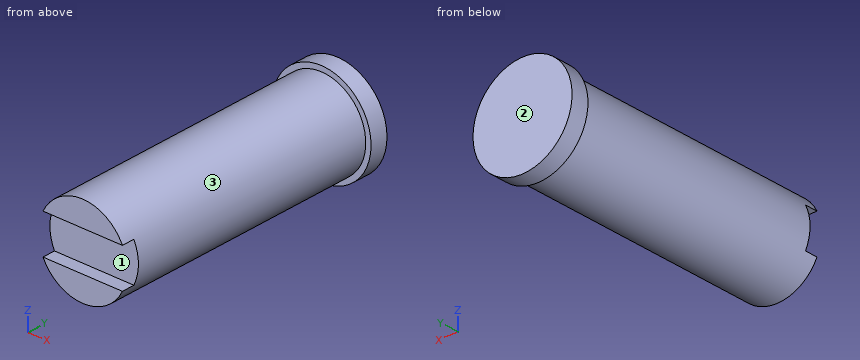
Autodesk Inventor part; units mm, degrees
ref_plane "YZ Plane" through (0, 0, 0) normal (1, 0, 0) x (0, 1, 0)
ref_plane "XZ Plane" through (0, 0, 0) normal (0, 1, 0) x (-1, 0, 0)
ref_plane "XY Plane" through (0, 0, 0) normal (0, 0, 1) x (1, 0, 0)
sketch "Sketch1" plane through (0, 0, 0) normal (0, 1, 0) x (-1, 0, 0)
  circle A0 centre (0, 0) radius 6.35
  dimension "d0" = 12.7
extrude "Extrusion1" add sketch "Sketch1" along normal blind 38.1
sketch "Sketch2" plane through (0, 38.1, 0) normal (0, 1, 0) x (1, 0, 0)
  circle A0 centre (0, 0) radius 7.112
  dimension "d3" = 14.224
extrude "Extrusion2" add sketch "Sketch2" along normal blind 2.54
sketch "Sketch3" plane through (0, 0, 0) normal (0, -1, 0) x (1, 0, 0)
  line L0 (-6.35, -2.794) -> (6.35, -2.794)
  line L1 (6.35, -2.794) -> (6.35, 2.794)
  line L2 (6.35, 2.794) -> (-6.35, 2.794)
  line L3 (-6.35, 2.794) -> (-6.35, -2.794)
  point P0 (0, 0)
  dimension "d6" = 5.588
extrude "Extrusion3" cut sketch "Sketch3" against normal blind 1.27
sketch "Sketch4" plane through (0, 1.27, 0) normal (0, -1, 0) x (1, 0, 0)
  point P0 (0, 0)
sketch "Sketch5" plane through (0, 1.27, 0) normal (0, -1, 0) x (1, 0, 0)
  line L0 (8.174, 2.794) -> (-7.6116, 2.794)
  line L1 (-7.6116, 2.794) -> (-7.6116, -2.794)
  line L2 (-7.6116, -2.794) -> (8.174, -2.794)
  line L3 (8.174, -2.794) -> (8.174, 2.794)
  point P0 (0, 0)
extrude "Extrusion4" cut sketch "Sketch5" against normal blind 0.5588
properties part number "key ejector"
Read the model definition and answer for the solid it produces. Units are mm, in the model's axes. Face numbers are marked on the shaded views. A direction names the side the tool comes from. Coordinates: 2 decimals unless noted, no trailing zeros. Order: outer loops, then holes, each group sorted by start corner. A loop starts at its lowest first (then second) coordinate and runs counter-clockwise, first axis right, second up. Notation, with made-up numbers: (21.25, -19.5) -> (47.25, -19.5) arc R31 cw to (47.25, 12.5) -> close; hole circle Ø11 at (19, 72). An arc over 180 degrees is marked (long way). Answer as a JSON object with one key per item and string values.
1) A cutting plane is placed at A-A, the plane z = 0. Determine the outline of the cut face in (x, y), plus the area to 3 significant figures.
Model answer:
{"outline": "(-7.11, 38.1) -> (-6.35, 38.1) -> (-6.35, 1.83) -> (6.35, 1.83) -> (6.35, 38.1) -> (7.11, 38.1) -> (7.11, 40.64) -> (-7.11, 40.64) -> close", "area": "497 mm²"}
2) Each of these flat-tipped pins is pushed along its axis until it touches: pin 1 (4.5 mm diameter, centred on x = -0.5, z = 0.5, fed in from -Y); pin 2 (2 mm diameter, centred on x = -2.5, y = 1, fed in from -Z); pin 3 (8 mm diameter, centred on x = 0.5, y = 30, fed in from -Z). Where does it stop, or does it pass through?
Model answer:
{"pin 1": "stops at y = 1.83", "pin 2": "stops at z = -6.17", "pin 3": "stops at z = -6.35"}
3) A cutting plane is placed at B-B, the plane x = 0. Determine the outline of the cut face in (y, z), plus the area to 3 significant figures.
Model answer:
{"outline": "(0, -6.35) -> (38.1, -6.35) -> (38.1, -7.11) -> (40.64, -7.11) -> (40.64, 7.11) -> (38.1, 7.11) -> (38.1, 6.35) -> (0, 6.35) -> (0, 2.79) -> (1.83, 2.79) -> (1.83, -2.79) -> (0, -2.79) -> close", "area": "510 mm²"}
4) Consider line 1 along Y through (x, z) = (-3.75, 5.25); line 2 along Y through (x, z) = (-2, -2.5); line 3 along X through (y, z) = (28, -5). Determine where each line is inside the solid, lowest interval first. Write a range as from..to.
Model answer:
{"line 1": "y = 38.1..40.64", "line 2": "y = 1.83..40.64", "line 3": "x = -3.91..3.91"}
5) A cutting plane is placed at D-D, the plane x = 4.5. Determine the outline of the cut face in (y, z), plus the area to 3 significant figures.
Model answer:
{"outline": "(0, -4.48) -> (38.1, -4.48) -> (38.1, -5.51) -> (40.64, -5.51) -> (40.64, 5.51) -> (38.1, 5.51) -> (38.1, 4.48) -> (0, 4.48) -> (0, 2.79) -> (1.83, 2.79) -> (1.83, -2.79) -> (0, -2.79) -> close", "area": "359 mm²"}
6) A cutting plane is placed at C-C, the plane y = 7. Determine the outline of the cut face in (x, z), plus the area to 3 significant figures.
Model answer:
{"outline": "circle Ø12.7 at (0, 0)", "area": "127 mm²"}
7) A tool of negligible diameter and unlimited length cuts with its end or side. For the marked faces 1, 2 and 3, from which of +Z, -Z, +X, -X, +Y, -Y can it reach the whole face along a straight path? Write none if from no direction.
Model answer:
{"face 1": "+X, -X, -Y", "face 2": "+Z, -Z, +X, -X, +Y", "face 3": "-Y"}
